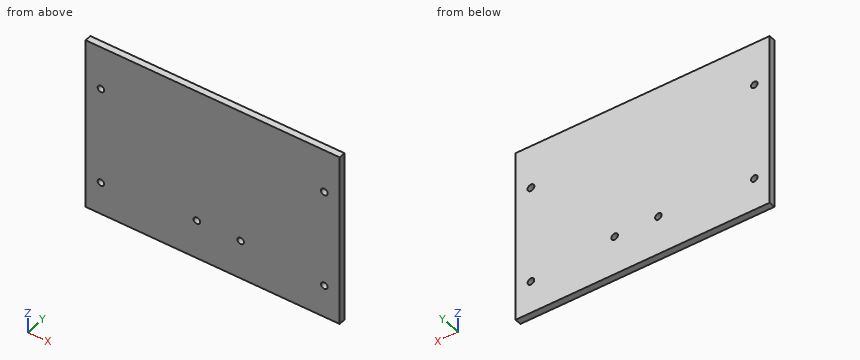
from build123d import *

# Parameters (mm, degrees)
SKETCH_1_W          = 116
SKETCH_1_H          = 80
EXTRUDE_1_DEPTH     = 3
SKETCH_2_R          = 1.5
SKETCH_2_R_2        = 1.55
CUT_EXTRUDE_1_DEPTH = 10
SKETCH_3_R          = 1.5
CUT_EXTRUDE_2_DEPTH = 71.519500849


with BuildPart() as part:
    # 草图1 → 凸台-拉伸1 (new body)
    with BuildSketch(Plane(origin=(0, 0, 0), x_dir=(1, 0, 0), z_dir=(0, 1, 0))):
        Rectangle(SKETCH_1_W, SKETCH_1_H)
    extrude(amount=EXTRUDE_1_DEPTH)

    # 草图2 → 切除-拉伸1 (cut)
    with BuildSketch(Plane.XZ):
        with Locations(Location((-51, 20, 0), (0, 0, 270))):
            Circle(SKETCH_2_R)
        with Locations(Location((51, 20, 0), (0, 0, 270))):
            Circle(SKETCH_2_R_2)
        with Locations(Location((51, -25, 0), (0, 0, 270))):
            Circle(SKETCH_2_R)
        with Locations(Location((-51, -25, 0), (0, 0, 270))):
            Circle(SKETCH_2_R)
    extrude(amount=-CUT_EXTRUDE_1_DEPTH, mode=Mode.SUBTRACT)

    # 草图3 → 切除-拉伸2 (cut, through all)
    with BuildSketch(Plane(origin=(0, 3, 0), x_dir=(1, 0, 0), z_dir=(0, 1, 0))):
        with Locations(Location((-7.215969028, 22, 0), (0, 0, 270))):
            Circle(SKETCH_3_R)
        with Locations(Location((12.784030972, 22, 0), (0, 0, 270))):
            Circle(SKETCH_3_R)
    extrude(amount=-CUT_EXTRUDE_2_DEPTH, mode=Mode.SUBTRACT)


solid = part.part
Source: CAD feature listing. Evaluate the final solid. Frame: model axes, mm. Coordinates: 2 decimals unless noted, no trailing zeros. Loops run counter-clockwise (first coordinate to the right, second up) from the corner with the lowest first, then second, coordinate; pieces in that order, holes last. Notation, with made-up numbers: (25.25, -33) - (75.25, -33) arc R8 cw to (75.25, -25) - close; hole circle Ø1 at (4.5, 85). An arc over 180 degrees is marked (long way). Return JSON: item names as keys, results as strings.
Q1. Section B-B, the plane x = 51. Return loops of the section in (y, z), plus the area to 3 significant figures.
Results:
{"outline": "(0, -40) - (3, -40) - (3, -26.5) - (0, -26.5) - close; (0, -23.5) - (3, -23.5) - (3, 18.45) - (0, 18.45) - close; (0, 21.55) - (3, 21.55) - (3, 40) - (0, 40) - close", "area": "222 mm2"}
Q2. Section A-A, the plane z = 20. Return loops of the section in (x, y).
Results:
{"outline": "(-58, 0) - (-52.5, 0) - (-52.5, 3) - (-58, 3) - close; (-49.5, 0) - (49.45, 0) - (49.45, 3) - (-49.5, 3) - close; (52.55, 0) - (58, 0) - (58, 3) - (52.55, 3) - close"}
Q3. Contact query for a flat-ended pin moving along its axis: P1, Ø4, axis at x = -7.22, z = -22, coming from the -Y side. Output: stop coordinate, or through.
Results:
{"P1": "y = 0"}
Q4. Material intervals for line 1 along X through (y, z) = (0.6, 20); line 2 along X through (y, z) = (1.4, -21), sorted ascending.
Results:
{"line 1": "-58 to -52.5, -49.5 to 49.45, 52.55 to 58", "line 2": "-58 to -8.33, -6.1 to 11.67, 13.9 to 58"}
